```python
from build123d import *

# Parameters (mm, degrees)
SKETCH1_W                      = 50
SKETCH1_H                      = 20
BASE_FLANGE1_DEPTH             = 2
EDGE_FLANGE1_STRIP_W           = 11.6
EDGE_FLANGE1_STRIP_H           = 2
EDGE_FLANGE1_STRIP_CUT_DEPTH   = 20
EDGE_FLANGE1_STRIP_2_W         = 11.6
EDGE_FLANGE1_STRIP_2_H         = 2
EDGE_FLANGE1_STRIP_CUT_2_DEPTH = 20
EDGE_FLANGE1_DEPTH             = 20
EDGE_FLANGE1_BEND_DEPTH        = 20


# Sheet-metal steps are written as plain solids
with BuildPart() as part:
    # Sketch1 → Base-Flange1 (new body)
    with BuildSketch(Plane.XY):
        with Locations((24.146981627, 10)):
            Rectangle(SKETCH1_W, SKETCH1_H)
    extrude(amount=-BASE_FLANGE1_DEPTH)

    # Edge-Flange1 strip (across the edge) → Edge-Flange1 strip cut (cut)
    with BuildSketch(Plane(origin=(-0.853018373, 0, -2), x_dir=(1, 0, 0), z_dir=(0, 1, 0))):
        with Locations((-2, -1)):
            Rectangle(EDGE_FLANGE1_STRIP_W, EDGE_FLANGE1_STRIP_H)
    extrude(amount=EDGE_FLANGE1_STRIP_CUT_DEPTH, mode=Mode.SUBTRACT)

    # Edge-Flange1 strip 2 (across the edge) → Edge-Flange1 strip cut 2 (cut)
    with BuildSketch(Plane(origin=(49.146981627, 20, -2), x_dir=(-1, 0, 0), z_dir=(0, -1, 0))):
        with Locations((-2, -1)):
            Rectangle(EDGE_FLANGE1_STRIP_2_W, EDGE_FLANGE1_STRIP_2_H)
    extrude(amount=EDGE_FLANGE1_STRIP_CUT_2_DEPTH, mode=Mode.SUBTRACT)

    # Edge-Flange1 section (across the edge) → Edge-Flange1 (add)
    with BuildSketch(Plane(origin=(-0.853018373, 0, -2), x_dir=(1, 0, 0), z_dir=(0, 1, 0))):
        with BuildLine():
            Line((0, 1.8), (0, 18))
            Line((0, 18), (2, 18))
            Line((2, 18), (2, 1.8))
            ThreePointArc((2, 1.8), (2.527207794, 0.527207794), (3.8, 0))
            Line((3.8, 0), (3.8, -2))
            ThreePointArc((3.8, -2), (1.112994231, -0.887005769), (0, 1.8))
        make_face()
    extrude(amount=EDGE_FLANGE1_DEPTH)

    # Edge-Flange1 section 2 (across the edge) → Edge-Flange1 bend (add)
    with BuildSketch(Plane(origin=(49.146981627, 20, -2), x_dir=(-1, 0, 0), z_dir=(0, -1, 0))):
        with BuildLine():
            Line((0, 1.8), (0, 18))
            Line((0, 18), (2, 18))
            Line((2, 18), (2, 1.8))
            ThreePointArc((2, 1.8), (2.527207794, 0.527207794), (3.8, 0))
            Line((3.8, 0), (3.8, -2))
            ThreePointArc((3.8, -2), (1.112994231, -0.887005769), (0, 1.8))
        make_face()
    extrude(amount=EDGE_FLANGE1_BEND_DEPTH)


solid = part.part
```
For this review, take the finished solid that the model builds, in its own axes (mm). A direction names the side the tool comes from. Give positions to 0.01 mm unless a question says otherwise; leave off trailing zeros. Write each loop counter-clockwise with the first axis right and the second up, starting at its lowest first coordinate (ties: lowest second). Pieces come first, ordered by that corner, then holes.
Item 1: Take a section at B-B (y = 2.25). Give the boundary of the cut face in (x, z).
Item 2: Insertion check: P1, Ø2, axis at x = 36.5, y = 11.5, coming from the -Z side; P2, Ø5, axis at x = 34, z = -6.5, coming from the +Y side. Each pin has a flat end and moves straight along its axis. Give the tip position at first contact, or say it passes through.
Item 3: Take a section at A-A (z = -14.5). Give the boundary of the cut face in (x, y), and give its area (3 significant figures).
Item 4: The part is to be moulded in two halves that separate along X. For faces 3 (the face through (46.63, 10.14, -2.54)), 4 (the face through (24, 0, -1)), 5 (the face through (-0.853, 10, -12)), 6 (the face through (48, 10.14, -1.08)), say which applies: +X half, -X half, draft (parallel to the pull), parting line (faces both ways), or undercut.
Item 5: Machinability: for faces 1 (the face through (48, 10, -20)), 2 (the face through (47.147, 10, -12)), which of the approach directions +Z, -Z, +X, -X, +Y, -Y give a long, thin tool a straight path to every point of the face, cutting with its end or side? Answer none if there is none.
Item 6: Take a section at C-C (x = 29). Give the boundary of the cut face in (y, z), and give its area (3 significant figures).
Item 7: Wall thickness on probe 1 along X at (y, z) = (16.75, -12); probe 2 along Z at (x, y) = (9.5, 5.5); probe 3 along Z at (x, y) = (2, 9.25): over which ranges is each line inside the solid? List them lowest first.
Established:
1. outline: (-0.85, -20) - (1.15, -20) - (1.15, -3.8) arc R1.8 cw to (2.95, -2) - (45.35, -2) arc R1.8 cw to (47.15, -3.8) - (47.15, -20) - (49.15, -20) - (49.15, -3.8) arc R3.8 ccw to (45.35, 0) - (2.95, 0) arc R3.8 ccw to (-0.85, -3.8) - close
2. P1: stops at z = -2
2. P2: passes through
3. outline: (-0.85, 0) - (1.15, 0) - (1.15, 20) - (-0.85, 20) - close; (47.15, 0) - (49.15, 0) - (49.15, 20) - (47.15, 20) - close
3. area: 80.0 mm2
4. face 3: undercut
4. face 4: draft
4. face 5: -X half
4. face 6: +X half
5. face 1: -Z, +X, -X, +Y, -Y
5. face 2: -Z, +Y, -Y
6. outline: (0, -2) - (20, -2) - (20, 0) - (0, 0) - close
6. area: 40.0 mm2
7. probe 1: x = -0.85 to 1.15, 47.15 to 49.15
7. probe 2: z = -2 to 0
7. probe 3: z = -2.27 to -0.12
